The listing builds one solid part. Answer for the finished solid, in the listing's coordinates (mm). Face numbers are marked on the shaded views. A direction names the side the tool comes from. Round coordinates to 2 decimals unless told otherwise and drop trailing zeros. Write each loop counter-clockwise with the first axis right and the second up, starting at its lowest first coordinate (ties: lowest second). Pieces come first, ordered by that corner, then holes. Notation, with made-up numbers: (25.5, 20) - (29.5, 20) arc R25 ccw to (29.5, 46) - close; hole circle Ø4 at (24, 62.25). An arc over 180 degrees is marked (long way). Use a Markdown table: item, result. Add a question column.
1) A cutting plane is placed at B-B (z = 9.25). Give the vertices of the cut face in (x, y).
2) A cutting plane is placed at C-C (y = -20.5). Give the vertices of the cut face in (x, z) (1 decimal), then the cut area to 3 significant figures.
3) A tool of negligible diameter and unlimited length cuts with its end or side. For the marked faces 1 and 2, from which of +Z, -Z, +X, -X, +Y, -Y can it reach the whole face along a straight path? Write none if from no direction.
4) Find the intervals of material crossed by probe 1 along Y at (x, z) = (-3, 9.75); probe 2 along X at (y, z) = (-46.5, 5); probe 3 along Y at (x, z) = (3, -2.5), in increasing order. Write a range as from..to.
5) Each of these flat-tipped pins is pushed along its axis until it touches: P1, Ø2, axis at x = -6.5, z = 0, coming from the -Y side; P2, Ø1, axis at x = -7.5, z = 9, coming from the +Y side; P3, Ø8, axis at x = 7, z = 5.5, coming from the +Y side; P4, Ø6, axis at x = 2, y = -65.5, coming from the -Z side. Where does it stop, or does it pass through?
6) A cutting plane is placed at A-A (x = 0). Give the vertices of the cut face in (y, z) (1 decimal), then the cut area to 3 significant figures.
7) A cutting plane is placed at D-D (z = -3). Give the vertices of the cut face in (x, y), then the cut area to 3 significant figures.
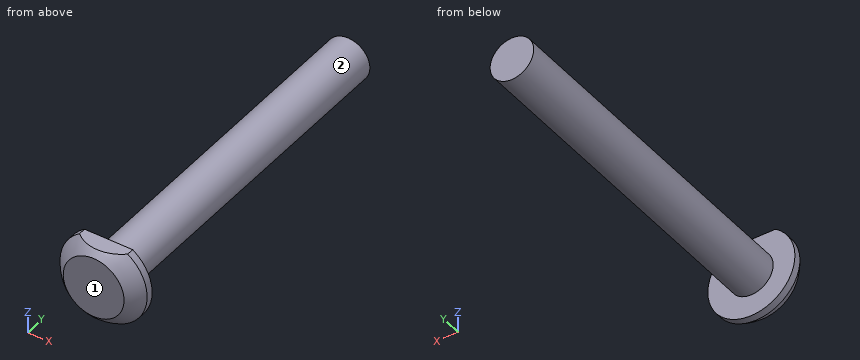
```python
from build123d import *

# Parameters (mm, degrees)
F0_R     = 4.7625
F1_DEPTH = 76.2
F2_R     = 9.525
F2_R_2   = 4.7625
F3_DEPTH = 1.5875
F7_DEPTH = 25.4


# Not quite as in the source:
# - a length typed as a fraction of an inch, garbled in the dataset ("3 / 203.2 mm" for 3/8 in), is restored


with BuildPart() as f1:
    # F0 (on Front) → F1 (new body)
    with BuildSketch(Plane.XZ):
        with Locations((0, 5.2942009643)):
            Circle(F0_R)
    extrude(amount=F1_DEPTH)

    # F2 (on face) → F3 (join)
    with BuildSketch(Plane.XZ.offset(76.2)):
        with Locations((0, 5.2942009643)):
            Circle(F2_R)
        with Locations((0, 5.2942009643)):
            Circle(F2_R_2, mode=Mode.SUBTRACT)
        with Locations((0, 5.2942009643)):
            Circle(F2_R_2)
    extrude(amount=F3_DEPTH)

    # F4 (on Right) → F5 (revolve)
    with BuildSketch(Plane.YZ):
        with BuildLine():
            ThreePointArc((-80.9625, -1.3615326297), (-79.514423226, -2.9504452476), (-77.7875, -4.2307990357))
            Line((-77.7875, -4.2307990357), (-77.7875, 5.2942009643))
            Line((-77.7875, 5.2942009643), (-80.9625, 5.2942009643))
            Line((-80.9625, 5.2942009643), (-80.9625, -1.3615326297))
        make_face()
    revolve(axis=Axis((0, -79.375, 5.2942009643), (0, 1, 0)))

    # F6 (on face) → F7 (cut)
    with BuildSketch(Plane(origin=(0, -76.2, 0), x_dir=(-1, 0, 0), z_dir=(0, 1, 0))):
        with BuildLine():
            Line((0, 13.2317009643), (5.2651418547, 13.2317009643))
            ThreePointArc((5.2651418547, 13.2317009643), (0, 14.8192009643), (-5.2651418547, 13.2317009643))
            Line((-5.2651418547, 13.2317009643), (0, 13.2317009643))
        make_face()
    extrude(amount=-F7_DEPTH, mode=Mode.SUBTRACT)


solid = f1.part
```
Entries:
| question | item | result |
|---|---|---|
| 1 | outline | (-8.66, -77.79) arc R10.38 ccw to (-5.35, -80.96) - (5.35, -80.96) arc R10.38 ccw to (8.66, -77.79) - (8.66, -76.2) - (2.65, -76.2) - (2.65, 0) - (-2.65, 0) - (-2.65, -76.2) - (-8.66, -76.2) - close |
| 2 | outline | circle Ø9.5 at (0, 5.3) |
| 2 | area | 71.3 mm² |
| 3 | face 1 | +Z, -Z, +X, -X, -Y |
| 3 | face 2 | +Y |
| 4 | probe 1 | y = -80.96..-76.2 |
| 4 | probe 2 | x = -4.75..4.75 |
| 4 | probe 3 | y = -79.39..-76.2 |
| 5 | P1 | stops at y = -80.37 |
| 5 | P2 | stops at y = -76.2 |
| 5 | P3 | stops at y = 0 |
| 5 | P4 | stops at z = 0.53 |
| 6 | outline | (-81, -1.4) arc R11.1 ccw to (-77.8, -4.2) - (-76.2, -4.2) - (-76.2, 0.5) - (0, 0.5) - (0, 10.1) - (-76.2, 10.1) - (-76.2, 13.2) - (-79.8, 13.2) arc R11.1 ccw to (-81, 11.9) - close |
| 6 | area | 804 mm² |
| 7 | outline | (-4.68, -77.79) arc R7.4 ccw to (4.68, -77.79) - (4.68, -76.2) - (-4.68, -76.2) - close |
| 7 | area | 25.6 mm² |
